Here's how the part is built. I have some questions about the finished solid (model axes, mm). A direction names the side the tool comes from. Round coordinates to 2 decimals unless told otherwise and drop trailing zeros. Write each loop counter-clockwise with the first axis right and the second up, starting at its lowest first coordinate (ties: lowest second). Pieces come first, ordered by that corner, then holes. Notation, with made-up numbers: (10.25, 9) - (14.25, 9) arc R28 ccw to (14.25, 39) - close; hole circle Ø3 at (67.25, 84). An arc over 180 degrees is marked (long way). Return JSON: item names as keys, results as strings. Group by question number.
```python
from build123d import *

# Parameters (mm, degrees)
F0_W     = 143.31
F0_H     = 35
F0_R     = 3.4
F0_R_2   = 5.15
F1_DEPTH = 14
F2_R     = 10
F2_R_2   = 5.15
F3_DEPTH = 6


with BuildPart() as f1:
    # F0 (on Top) → F1 (new body)
    with BuildSketch(Plane.XY):
        with Locations((0, 2.5)):
            Rectangle(F0_W, F0_H)
        with Locations((-62.155, 0)):
            Circle(F0_R, mode=Mode.SUBTRACT)
        with Locations((62.155, 0)):
            Circle(F0_R, mode=Mode.SUBTRACT)
        Polygon((-10, 55), (-71.655, 20), (71.655, 20), (10, 55), align=None)
        with Locations((0, 36)):
            Circle(F0_R_2, mode=Mode.SUBTRACT)
    extrude(amount=F1_DEPTH)

    # F2 (on face) → F3 (join)
    with BuildSketch(Plane(origin=(0, 0, 0), x_dir=(1, 0, 0), z_dir=(0, 0, -1))):
        with Locations((0, -36)):
            Circle(F2_R)
        with Locations((0, -36)):
            Circle(F2_R_2, mode=Mode.SUBTRACT)
    extrude(amount=F3_DEPTH)


solid = f1.part
```
1) If we mould it in two halves opening along Y, with no side actions, what happens to faces 1 (the flat face through (-1, -15, 7)), 2 (the flat face through (-5, 34, -6)), 3 (the cylindrical face through (-59.014, -1.302, 6.902))? For each: released by +Y, released by -Y, zero draft, split by the parting line, or undercut.
2) Imagine slicing it at C-C (y = 36). Please give me the cut outline in (x, z), plus the area to 3 significant figures.
3) Imagine slicing it at D-D (x = 7.5). Please give me the cut outline in (y, z), plus the area to 3 significant figures.
4) I need wall thicknesses on line 1 along X through (y, z) = (3, 7.25) (3 decimals); line 2 along X through (y, z) = (-0.5, 9.5) (3 decimals); line 3 along Z through (x, y) = (-18, 0). Which ranges of each line are inside material? Lowest first, please.
5) Imagine slicing it at B-B (z = 9.5). Please give me the cut outline in (x, y) (3 decimals), plus the area to 3 significant figures.
6) Will these pins go through, and if not, where does the flat tip stop? pin 1 Ø6 at (y, z) = (28.5, 0) entering from +X; pin 2 Ø1.5 at (x, z) = (-19.5, 10) entering from +Y; pin 3 Ø1.5 at (x, y) = (-15.5, 45.5) entering from -Z.
7) Imagine slicing it at A-A (y = 0). Please give me the cut outline in (x, z) (3 decimals), plus the area to 3 significant figures.
8) For faces 4 (the cylindrical face through (-2.17, 45.76, -2.96)), 5 (the flat face through (-1, 13, 14)), which set-ups out of +Z, -Z, +X, -X, +Y, -Y let a thin tool reach every point of the face, with its end or its side?
Results found:
{
 "1": {"face 1": "released by -Y", "face 2": "zero draft", "face 3": "undercut"},
 "2": {"outline": "(-43.47, 0) - (-10, 0) - (-10, -6) - (-5.15, -6) - (-5.15, 14) - (-43.47, 14) - close; (5.15, -6) - (10, -6) - (10, 0) - (43.47, 0) - (43.47, 14) - (5.15, 14) - close", "area": "1,130 mm²"},
 "3": {"outline": "(-15, 0) - (29.39, 0) - (29.39, -6) - (42.61, -6) - (42.61, 0) - (55, 0) - (55, 14) - (-15, 14) - close", "area": "1,060 mm²"},
 "4": {"line 1": "x = -71.655 to -63.755, -60.555 to 60.555, 63.755 to 71.655", "line 2": "x = -71.655 to -65.518, -58.792 to 58.792, 65.518 to 71.655", "line 3": "z = 0 to 14"},
 "5": {"outline": "(-71.655, -15) - (71.655, -15) - (71.655, 20) - (10, 55) - (-10, 55) - (-71.655, 20) - close; hole circle Ø6.8 at (-62.155, 0); hole circle Ø10.3 at (0, 36); hole circle Ø6.8 at (62.155, 0)", "area": "7,720 mm²"},
 "6": {"pin 1": "stops at x = 61.97", "pin 2": "stops at y = 50.03", "pin 3": "stops at z = 0"},
 "7": {"outline": "(-71.655, 0) - (-65.555, 0) - (-65.555, 14) - (-71.655, 14) - close; (-58.755, 0) - (58.755, 0) - (58.755, 14) - (-58.755, 14) - close; (65.555, 0) - (71.655, 0) - (71.655, 14) - (65.555, 14) - close", "area": "1,820 mm²"},
 "8": {"face 4": "-Z", "face 5": "+Z, +X, -X, +Y, -Y"}
}
